Could you check a few things on this model? Use its own coordinates, in mm. A direction names the side the tool comes from. Give positions to 0.01 mm unless a question says otherwise; leave off trailing zeros. Order: outer loops, then holes, each group sorted by start corner. A loop starts at its lowest first (then second) coordinate and runs counter-clockwise, first axis right, second up. Notation, with made-up numbers: (-36, 66) -> (-3, 66) arc R21 cw to (-3, 80) -> close; hole circle Ø4 at (76, 21.25). An arc over 180 degrees is marked (long way). Write each question's results on one line, items separated by ' | '.
Autodesk Inventor part; units mm, degrees
ref_plane "YZ Plane" through (0, 0, 0) normal (1, 0, 0) x (0, 1, 0)
ref_plane "XZ Plane" through (0, 0, 0) normal (0, 1, 0) x (-1, 0, 0)
ref_plane "XY Plane" through (0, 0, 0) normal (0, 0, 1) x (1, 0, 0)
sketch "Sketch1" plane through (0, 0, 0) normal (0, 0, 1) x (1, 0, 0)
  line L0 (0, 0) -> (2.5, 0)
  line L1 (2.5, 0) -> (2.5, 35)
  line L2 (2.5, 35) -> (-2.5, 35)
  line L3 (-2.5, 35) -> (-2.5, 0)
  circle A0 centre (0, 0) radius 8.5
  line L4 (0, 35) -> (8.5, 35) construction
  circle A1 centre (0, 35) radius 8.5
  line L5 (-8.5, 0) -> (-8.5, 35)
  line L6 (8.5, 35) -> (8.5, 0)
  line L7 (0, 35) -> (8.5, 35)
  line L8 (0, 35) -> (-8.5, 26.5)
  line L9 (0, 35) -> (12.0208, 35) construction
  line L10 (0, 0) -> (8.5, 0)
  line L11 (0, 0) -> (-8.5, 8.5)
  line L12 (0, 0) -> (12.0208, 0) construction
  dimension "d9" = 17
  dimension "d1" = 2.5
  dimension "d2" = 35
  dimension "d3" = 5
  dimension "d5" = 17
  dimension "d10" = 2.5
  dimension "d11" = 0
  dimension "d12" = 135
  dimension "d13" = 135
extrude "Extrusion1" add sketch "Sketch1" along normal blind 20 contours L11 L3 A0 L1 L0 | L1 A0 L10 | L11 A0 L3 | A0 L3 A1 L1 | L1 A1 L6 A0 | A0 L11 L5 L8 A1 L3 | A1 L3 L8 L2 L1 | L1 L7 A1 | A1 L8 L3
sketch "Sketch2" plane through (0, 0, 0) normal (0, 0, -1) x (-1, 0, 0)
  line L0 (0, 0) -> (-8.5, 0)
  line L1 (0, 0) -> (0, 8)
  circle A0 centre (0, 8) radius 2.5
  line L2 (8.5, 8.5) -> (0, 0)
  line L3 (0, 0) -> (-1.5, 0)
  line L4 (-1.5, 0) -> (-1.5, 8)
  line L5 (-1.5, 8) -> (1.5, 8)
  line L6 (1.5, 8) -> (1.5, 0)
  line L7 (1.5, 0) -> (0, 0)
  line L8 (0, 35) -> (8.5, 26.5)
  line L9 (0, 35) -> (0, 27)
  line L10 (0, 27) -> (-1.5, 27)
  line L11 (-1.5, 27) -> (-1.5, 35)
  line L12 (-8.5, 35) -> (0, 35)
  line L13 (0, 27) -> (1.5, 27)
  line L14 (1.5, 27) -> (1.5, 35)
  line L15 (1.5, 35) -> (0, 35)
  circle A1 centre (0, 27) radius 2.5
  point P0 (1.5, 45)
  point P1 (-1.5, 29)
  point P2 (1.5, 29)
  point P3 (-1.5, 6)
  point P4 (1.5, 6)
  dimension "d16" = 8
  dimension "d17" = 5
  dimension "d18" = 1.5
  dimension "d19" = 3
  dimension "d20" = 8
  dimension "d21" = 1.5
  dimension "d22" = 1.5
  dimension "d23" = 5
extrude "Extrusion2" cut sketch "Sketch2" against normal through all
fillet "Fillet1" radius 8 4 edges at (8.5, 17.5, 0) (8.5, 17.5, 20) (-8.5, 17.5, 0) (-8.5, 17.5, 20)
sketch "Sketch4" plane through (1.5, 0, 0.0627) normal (0, -1, 0) x (1, 0, 0)
  line L0 (-10, 7.9373) -> (-10, 11.9373)
  line L1 (-10, 9.9373) -> (-8, 9.9373)
  circle A0 centre (-8, 9.9373) radius 1
  point P0 (-1.5, -0.0627)
  dimension "d31" = 2
  dimension "d32" = 2
extrude "Extrusion4" cut sketch "Sketch4" against normal through all
properties part number "pinky_f1"
Q1. I'm going to push flat-ended pins straight in: pin 1 Ø4 at (y, z) = (30, 3) entering from +X; pin 2 Ø5 at (y, z) = (2.5, 12.5) entering from -X; pin 3 Ø1.6 at (x, z) = (-6.5, 10) entering from +Y; pin 4 Ø1 at (x, y) = (-5, 12) entering from +Z. Where does each tip first touch, or does it pass through?
Here are the results:
pin 1: stops at x = 7.92 | pin 2: stops at x = -5 | pin 3: passes through | pin 4: stops at z = 18.93
Q2. Suppose I cut it at C-C on x = -2. Please give me the cut outline in (y, z), and give its area (3 significant figures).
Here are the results:
outline: (2, 0.14) -> (6.5, 0.14) -> (6.5, 19.86) -> (2, 19.86) -> close; (9.5, 0.14) -> (25.5, 0.14) -> (25.5, 19.86) -> (9.5, 19.86) -> close; (28.5, 0.14) -> (33, 0.14) -> (33, 19.86) -> (28.5, 19.86) -> close | area: 493 mm²
Q3. For faces 1 (the flat face through (-1.5, 4, 10)), 2 (the flat face through (-1.5, 31, 10)), 3 (the flat face through (4, 35, 10)), which set-ups out of +Z, -Z, +X, -X, +Y, -Y let a thin tool reach every point of the face, with its end or its side?
Here are the results:
face 1: +Z, -Z, -Y | face 2: +Z, -Z, +Y | face 3: +Z, -Z, +X, -X, +Y
Q4. I need wall thicknesses on line 1 along X through (y, z) = (27, 10.75); line 2 along Y through (x, z) = (-0.5, 15.25); line 3 along X through (y, z) = (22.75, 10). Which ranges of each line are inside material? Lowest first, please.
Here are the results:
line 1: x = -8 to -7.16, -5.84 to -2.5, 2.5 to 8.5 | line 2: y = 10.45 to 24.55 | line 3: x = -8.5 to -7.5, -5.5 to 8.5
Q5. Thinking about a two-plate mould opening in Z: for faces 4 (the flat face through (0, 18, 0)), 5 (the flat face through (8.5, 18, 10)), 6 (the cylindrical face through (-5.546, 17.332, 10.3)), which applies, +Z half, -Z half, draft (parallel to the pull), parting line (faces both ways), or undercut?
Here are the results:
face 4: -Z half | face 5: draft | face 6: undercut
Q6. Suppose I cut it at D-D on y = 12.5. Please give me the cut outline in (x, z), and give its area (3 significant figures).
Here are the results:
outline: (-8.5, 8) arc R8 ccw to (-0.5, 0) -> (0.5, 0) arc R8 ccw to (8.5, 8) -> (8.5, 12) arc R8 ccw to (0.5, 20) -> (-0.5, 20) arc R8 ccw to (-8.5, 12) -> close; hole circle Ø2 at (-6.5, 10) | area: 282 mm²
Q7. Suppose I cut it at A-A on z = 10. Please give me the cut outline in (x, y).
Here are the results:
outline: (-8.5, 8.5) -> (-7.5, 7.5) -> (-7.5, 27.5) -> (-8.5, 26.5) -> close; (-5.5, 5.5) -> (-1.5, 1.5) -> (-1.5, 6) arc R2.5 cw (long way) to (1.5, 6) -> (1.5, 0) -> (8.5, 0) -> (8.5, 35) -> (1.5, 35) -> (1.5, 29) arc R2.5 cw (long way) to (-1.5, 29) -> (-1.5, 33.5) -> (-5.5, 29.5) -> close
Q8. Suppose I cut it at B-B on y = 27. Please give me the cut outline in (x, z), and give its area (3 significant figures).
Here are the results:
outline: (-8, 5.22) arc R8 ccw to (-2.5, 0.25) -> (-2.5, 19.75) arc R8 ccw to (-8, 14.78) -> close; (2.5, 0.25) arc R8 ccw to (8.5, 8) -> (8.5, 12) arc R8 ccw to (2.5, 19.75) -> close; hole circle Ø2 at (-6.5, 10) | area: 179 mm²
